Model file for the job. Use its own axes, mm. A direction names the side the tool comes from. Round coordinates to 2 decimals unless told otherwise and drop trailing zeros. Loops run counter-clockwise (first coordinate to the right, second up) from the corner with the lowest first, then second, coordinate; pieces in that order, holes last. Notation, with made-up numbers: M -13,15.25 L 16,15.25 A37 ccw 16,52.25 Z; hole C 37.25,52.5 d10. An arc over 180 degrees is marked long. Use a Markdown table: item, result. Add a question column.
Item 1: Saw through at A-A on y = 4.5. Write the cut outline in (x, z), then the cut area to 3 significant figures.
Item 2: Two-plate mould, pull along X, no slides. Class faces 6 (the cylindrical face through (0.059, -6.946, 0.674)), 7 (the flat face through (-2, -2, 0)), 8 (the flat face through (-4.725, -2.786, 0.656)): +X half, -X half, draft (parallel to the pull), parting line (faces both ways), or undercut.
Item 3: Wall check: L1, parallel to Y at x = 0, z = 1; L2, parallel to Y at x = 0, z = 1.2; L3, parallel to X at y = -6.5, z = 0.95. Give the ranges that are in metal, low to high. Write a range as from..to.
Item 4: Saw through at B-B on x = -6.5. Write the cut outline in (y, z).
Item 5: Tool access for faces 1 (the cylindrical face through (-1.825, -1.4, 2.464)), 2 (the flat face through (1.9, 5, 1)), 3 (the flat face through (-1.9, 5, 1)), 4 (the flat face through (-1, -1, 1.1)), 5 (the flat face through (1.9, -5, 1)): list every direction of +Z, -Z, +X, -X, +Y, -Y with a clear straight run to the whole face (end or side of a thin tool).
Item 6: Saw through at C-C on y = 0. Give the number of separate pieces and of enclosed holes in the cut face, then the cut area to 3 significant figures.
Item 7: Pin check, flat tips, straight feed: P1, Ø1.4, axis at x = -1, y = -0.5, coming from the +Z side; P2, Ø1.5, axis at y = 4.5, z = 0.5, coming from the -X side; P3, Ø1.1, axis at y = -4.5, z = 0.5, coming from the +X side. Stop position of each tip, or through.
```python
from build123d import *

# Parameters (mm, degrees)
AUFSATZ_LINEAR_AUSTRAGEN1_DEPTH      = 1.33
AUFSATZ_LINEAR_AUSTRAGEN2_DEPTH      = 2.3
AUFSATZ_LINEAR_AUSTRAGEN2_DEPTH_BACK = 1.33
SKIZZE2_R                            = 3.4
SKIZZE2_R_2                          = 2.3
SKIZZE3_R                            = 1.25
SCHNITT_LINEAR_AUSTRAGEN1_DEPTH      = 21.470115412
SKIZZE4_R                            = 2.35
SCHNITT_LINEAR_AUSTRAGEN2_DEPTH      = 1.1
SKIZZE5_R                            = 0.45
SCHNITT_LINEAR_AUSTRAGEN3_DEPTH      = 21.470115412
SCHNITT_LINEAR_AUSTRAGEN4_DEPTH      = 1.33


with BuildPart() as part:
    # Skizze1 → Aufsatz-Linear austragen1 (new body)
    with BuildSketch(Plane.XY):
        with BuildLine():
            Line((-16.79191458, 1.869621687), (-1.9, 3))
            Line((-1.9, 3), (-1.9, 6.5))
            ThreePointArc((-1.9, 6.5), (0, 8.4), (1.9, 6.5))
            Line((1.9, 6.5), (1.9, 3))
            Line((1.9, 3), (16.79191458, 1.869621687))
            ThreePointArc((16.79191458, 1.869621687), (18.525, 0), (16.79191458, -1.869621687))
            Line((16.79191458, -1.869621687), (1.9, -3))
            Line((1.9, -3), (1.9, -6.5))
            ThreePointArc((1.9, -6.5), (0, -8.4), (-1.9, -6.5))
            Line((-1.9, -6.5), (-1.9, -3))
            Line((-1.9, -3), (-16.79191458, -1.869621687))
            ThreePointArc((-16.79191458, -1.869621687), (-18.525, 0), (-16.79191458, 1.869621687))
        make_face()
    extrude(amount=AUFSATZ_LINEAR_AUSTRAGEN1_DEPTH)

    # Skizze2 → Aufsatz-Linear austragen2 (add, two sides: drawn at the far end of the back side and taken through both)
    with BuildSketch(Plane.XY.offset(1.33).offset(-AUFSATZ_LINEAR_AUSTRAGEN2_DEPTH_BACK)):
        Circle(SKIZZE2_R)
        Circle(SKIZZE2_R_2, mode=Mode.SUBTRACT)
    extrude(amount=AUFSATZ_LINEAR_AUSTRAGEN2_DEPTH + AUFSATZ_LINEAR_AUSTRAGEN2_DEPTH_BACK)

    # Skizze3 → Schnitt-Linear austragen1 (cut, through all)
    with BuildSketch(Plane.XY.offset(1.33)):
        Circle(SKIZZE3_R)
    extrude(amount=-SCHNITT_LINEAR_AUSTRAGEN1_DEPTH, mode=Mode.SUBTRACT)

    # Skizze4 → Schnitt-Linear austragen2 (cut)
    with BuildSketch(Plane(origin=(0, 0, 0), x_dir=(-1, 0, 0), z_dir=(0, 0, -1))):
        Circle(SKIZZE4_R)
    extrude(amount=-SCHNITT_LINEAR_AUSTRAGEN2_DEPTH, mode=Mode.SUBTRACT)

    # Skizze5 → Schnitt-Linear austragen3 (cut, through all)
    with BuildSketch(Plane.XY.offset(1.33)):
        with Locations((0, 6.5)):
            Circle(SKIZZE5_R)
        with Locations((-16.65, 0)):
            Circle(SKIZZE5_R)
        with Locations((0, 4.5)):
            Circle(SKIZZE5_R)
        with Locations((-14.65, 0)):
            Circle(SKIZZE5_R)
        with Locations((-12.65, 0)):
            Circle(SKIZZE5_R)
        with Locations((-10.65, 0)):
            Circle(SKIZZE5_R)
        with Locations((-8.65, 0)):
            Circle(SKIZZE5_R)
        with Locations((-6.65, 0)):
            Circle(SKIZZE5_R)
        with Locations((-4.65, 0)):
            Circle(SKIZZE5_R)
        with Locations(Location((0, -4.5, 0), (0, 0, 180))):
            Circle(SKIZZE5_R)
        with Locations(Location((0, -6.5, 0), (0, 0, 180))):
            Circle(SKIZZE5_R)
        with Locations(Location((4.65, 0, 0), (0, 0, 180))):
            Circle(SKIZZE5_R)
        with Locations(Location((6.65, 0, 0), (0, 0, 180))):
            Circle(SKIZZE5_R)
        with Locations(Location((8.65, 0, 0), (0, 0, 180))):
            Circle(SKIZZE5_R)
        with Locations(Location((10.65, 0, 0), (0, 0, 180))):
            Circle(SKIZZE5_R)
        with Locations(Location((12.65, 0, 0), (0, 0, 180))):
            Circle(SKIZZE5_R)
        with Locations(Location((14.65, 0, 0), (0, 0, 180))):
            Circle(SKIZZE5_R)
        with Locations(Location((16.65, 0, 0), (0, 0, 180))):
            Circle(SKIZZE5_R)
    extrude(amount=-SCHNITT_LINEAR_AUSTRAGEN3_DEPTH, mode=Mode.SUBTRACT)

    # Skizze6 → Schnitt-Linear austragen4 (cut)
    with BuildSketch(Plane(origin=(0, 0, 0), x_dir=(-1, 0, 0), z_dir=(0, 0, -1))):
        Polygon((-7.630661654, -0.069500342), (-7.630661654, 5.641889325), (-18.981826271, 5.641889325), (-18.981826271, -4.018658181), (-7.630661654, -4.018658181), align=None)
        Polygon((7.630661654, -4.018658181), (7.630661654, -0.069500342), (7.630661654, 5.641889325), (18.981826271, 5.641889325), (18.981826271, -4.018658181), align=None)
    extrude(amount=-SCHNITT_LINEAR_AUSTRAGEN4_DEPTH, mode=Mode.SUBTRACT)


solid = part.part
```
Entries:
| question | item | result |
|---|---|---|
| 1 | outline | M -1.9,0 L -0.45,0 L -0.45,1.33 L -1.9,1.33 Z; M 0.45,0 L 1.9,0 L 1.9,1.33 L 0.45,1.33 Z |
| 1 | area | 3.86 mm2 |
| 2 | face 6 | undercut |
| 2 | face 7 | draft |
| 2 | face 8 | -X half |
| 3 | L1 | -8.4..-6.95, -6.05..-4.95, -4.05..-2.35, 2.35..4.05, 4.95..6.05, 6.95..8.4 |
| 3 | L2 | -8.4..-6.95, -6.05..-4.95, -4.05..-1.25, 1.25..4.05, 4.95..6.05, 6.95..8.4 |
| 3 | L3 | -1.9..-0.45, 0.45..1.9 |
| 4 | outline | M -2.65,0 L -0.42,0 L -0.42,1.33 L -2.65,1.33 Z; M 0.42,0 L 2.65,0 L 2.65,1.33 L 0.42,1.33 Z |
| 5 | face 1 | +Z |
| 5 | face 2 | +Z, -Z, +X, +Y |
| 5 | face 3 | +Z, -Z, -X, +Y |
| 5 | face 4 | -Z |
| 5 | face 5 | +Z, -Z, +X, -Y |
| 6 | separate pieces | 6 |
| 6 | enclosed holes | 0 |
| 6 | area | 14.8 mm2 |
| 7 | P1 | z = 1.33 |
| 7 | P2 | x = -1.9 |
| 7 | P3 | x = 1.9 |
